```python
from build123d import *

# Parameters (mm, degrees)
ESBO_O1_R                = 20
RESSALTO_EXTRUS_O1_DEPTH = 3
ESBO_O2_W                = 4
ESBO_O2_H                = 8
ESBO_O2_R                = 1
RESSALTO_EXTRUS_O3_DEPTH = 4.5
ESBO_O3_W                = 23
ESBO_O3_H                = 13
CORTE_EXTRUS_O1_DEPTH    = 1
ESBO_O4_W                = 28
ESBO_O4_H                = 5
RESSALTO_EXTRUS_O4_DEPTH = 15


with BuildPart() as part:
    # Esboço1 → Ressalto-extrusão1 (new body)
    with BuildSketch(Plane.XY):
        Circle(ESBO_O1_R)
        with BuildLine():
            ThreePointArc((5.921389022, 2.680886429), (-6.5, 0), (5.921389022, -2.680886429))
            ThreePointArc((5.921389022, -2.680886429), (9.242616034, 0), (5.921389022, 2.680886429))
        make_face(mode=Mode.SUBTRACT)
    extrude(amount=RESSALTO_EXTRUS_O1_DEPTH)

    # Esboço2 → Ressalto-extrusão3 (add)
    with BuildSketch(Plane.XY.offset(3)):
        with Locations((-8.5, 0)):
            Rectangle(ESBO_O2_W, ESBO_O2_H)
        with Locations((-8.5, 0)):
            Circle(ESBO_O2_R, mode=Mode.SUBTRACT)
        with BuildLine():
            Line((16.5, -4), (19.595917942, -4))
            ThreePointArc((19.595917942, -4), (20, 0), (19.595917942, 4))
            Line((19.595917942, 4), (16.5, 4))
            Line((16.5, 4), (16.5, -4))
        make_face()
        with Locations((18.5, 0)):
            Circle(ESBO_O2_R, mode=Mode.SUBTRACT)
    extrude(amount=RESSALTO_EXTRUS_O3_DEPTH)

    # Esboço3 → Corte-extrusão1 (cut)
    with BuildSketch(Plane.XY.offset(3)):
        with Locations((5, 0)):
            Rectangle(ESBO_O3_W, ESBO_O3_H)
    extrude(amount=-CORTE_EXTRUS_O1_DEPTH, mode=Mode.SUBTRACT)

    # Esboço4 → Ressalto-extrusão4 (add)
    with BuildSketch(Plane.XY.offset(3)):
        with Locations((0, -11.5)):
            Rectangle(ESBO_O4_W, ESBO_O4_H)
    extrude(amount=RESSALTO_EXTRUS_O4_DEPTH)


solid = part.part
```
Geometry: final body of the model. Coordinates: model frame, mm. A direction names the side the tool comes from. Give positions to 0.01 mm unless a question says otherwise; leave off trailing zeros. Write each loop counter-clockwise with the first axis right and the second up, starting at its lowest first coordinate (ties: lowest second). Pieces come first, ordered by that corner, then holes.
1. Line query: probe 1 along Y at (x, z) = (-8.5, 5.95); probe 2 along Y at (x, z) = (18.5, 4.4); probe 3 along Y at (x, z) = (0, 1.4). Output: solid intervals per line, ascending.
2. Section query C-C, the plane x = 5. Return loops of the section in (y, z).
3. Draft query along Y for faces 4 (the cylindrical face through (19.87, 2.27, 2.03)), 5 (the flat face through (12, 0, 2)), 6 (the flat face through (-10.5, 0, 5)). Return one class per face: released by +Y, released by -Y, zero draft, split by the parting line, or undercut.
4. Section query D-D, the plane x = 18.5. Return loops of the section in (y, z), then the cut area to 3 significant figures.
5. Pin query (flat end, axial travel): P1, Ø11.5, axis at x = 0, y = 0, coming from the -Z side; P2, Ø10, axis at x = -11, y = -10.5, coming from the -Z side; P3, Ø1.6, axis at x = -8.5, y = -0.5, coming from the +Z side; P4, Ø0.9, axis at x = 18, z = 5.5, coming from the +Y side. Return the tip coordinate at first contact, or that it passes through.
6. Section query A-A, the plane z = 7. Return loops of the section in (x, y).
7. Section query B-B, the plane y = 5. Return loops of the section in (x, z).
8. Reachability of faces 1 (the flat face through (18, 4, 5)), 2 (the flat face through (18, -4, 5)), 3 (the flat face through (-9, 0, 3)) from +Z, -Z, +X, -X, +Y, -Y: full face, straight path, thin tool, end or side. Return the list, or none.
Computed:
1. probe 1: y = -14 to -9, -4 to -1, 1 to 4
1. probe 2: y = -4 to -1, 1 to 4
1. probe 3: y = -20 to -6.5, 6.5 to 20
2. outline: (-19.36, 0) - (-4.15, 0) - (-4.15, 2) - (-6.5, 2) - (-6.5, 3) - (-9, 3) - (-9, 18) - (-14, 18) - (-14, 3) - (-19.36, 3) - close; (4.15, 0) - (19.36, 0) - (19.36, 3) - (6.5, 3) - (6.5, 2) - (4.15, 2) - close
3. face 4: split by the parting line
3. face 5: undercut
3. face 6: zero draft
4. outline: (-7.6, 0) - (7.6, 0) - (7.6, 3) - (4, 3) - (4, 7.5) - (1, 7.5) - (1, 3) - (-1, 3) - (-1, 7.5) - (-4, 7.5) - (-4, 3) - (-7.6, 3) - close
4. area: 72.6 mm2
5. P1: passes through
5. P2: stops at z = 0
5. P3: stops at z = 7.5
5. P4: stops at y = 4
6. outline: (-14, -14) - (14, -14) - (14, -9) - (-14, -9) - close; (-10.5, -4) - (-6.5, -4) - (-6.5, 4) - (-10.5, 4) - close; (16.5, -4) - (19.6, -4) arc R20 ccw to (19.6, 4) - (16.5, 4) - close; hole circle Ø2 at (-8.5, 0); hole circle Ø2 at (18.5, 0)
7. outline: (-19.36, 0) - (-4.15, 0) - (-4.15, 2) - (-6.5, 2) - (-6.5, 3) - (-19.36, 3) - close; (4.15, 0) - (19.36, 0) - (19.36, 3) - (16.5, 3) - (16.5, 2) - (4.15, 2) - close
8. face 1: +Z, +X, -X, +Y
8. face 2: +Z, +X, -X, -Y
8. face 3: +Z
